Geometry: final body of the model. Coordinates: model frame, mm. A direction names the side the tool comes from. Round coordinates to 2 decimals unless told otherwise and drop trailing zeros. Loops run counter-clockwise (first coordinate to the right, second up) from the corner with the lowest first, then second, coordinate; pieces in that order, holes last. Notation, with made-up numbers: (-5, -13) - (31, -13) arc R16 cw to (31, 18) - close; hole circle Ø3 at (85, -19). An arc over 180 degrees is marked (long way). Answer as CSV lines item,"result".
from build123d import *

# Parameters (mm, degrees)
SKETCH1_R           = 0.899918091
SKETCH1_R_2         = 0.899925125
SKETCH1_R_3         = 1.45
SKETCH1_R_4         = 8
SKETCH1_W           = 3.400011
SKETCH1_H           = 6.2
SKETCH1_W_2         = 3.4
BOSS_EXTRUDE2_DEPTH = 5.85


with BuildPart() as part:
    # Sketch1 → Boss-Extrude2 (new body)
    with BuildSketch(Plane.XY):
        with BuildLine():
            Line((669.21684417, 349.14615334), (647.916445931, 349.14615334))
            ThreePointArc((647.916445931, 349.14615334), (647.089176563, 348.803487148), (646.746510371, 347.976217781))
            Line((646.746510371, 347.976217781), (646.746510371, 315.835342781))
            add(Edge.make_bspline(
                [(646.746510371, 315.835342781), (646.746510371, 314.02716752), (648.773268796, 314.14615334)],
                knots=[0, 0, 0, 1, 1, 1], degree=2))
            Line((648.773268796, 314.14615334), (669.21684417, 314.14615334))
            Line((669.21684417, 314.14615334), (683.493527466, 314.14615334))
            ThreePointArc((683.493527466, 314.14615334), (688.18557682, 319.867900287), (681.655729571, 323.348533873))
            ThreePointArc((681.655729571, 323.348533873), (669.218799175, 331.833597772), (681.99878285, 339.792590441))
            ThreePointArc((681.99878285, 339.792590441), (688.860665305, 343.178948939), (684.070537296, 349.14615334))
            Line((684.070537296, 349.14615334), (669.21684417, 349.14615334))
        make_face()
        with Locations((684.726521371, 342.89615334)):
            Circle(SKETCH1_R, mode=Mode.SUBTRACT)
        with Locations((684.726521371, 320.39615334)):
            Circle(SKETCH1_R_2, mode=Mode.SUBTRACT)
        with Locations((658.726521371, 319.24615334)):
            Circle(SKETCH1_R_3, mode=Mode.SUBTRACT)
        with Locations((658.726521371, 331.64615334)):
            Circle(SKETCH1_R_4, mode=Mode.SUBTRACT)
        with Locations((651.446515871, 343.04615334)):
            Rectangle(SKETCH1_W, SKETCH1_H, mode=Mode.SUBTRACT)
        with Locations((653.576521371, 319.24615334)):
            Rectangle(SKETCH1_W_2, SKETCH1_H, mode=Mode.SUBTRACT)
        with Locations((666.006526871, 343.04615334)):
            Rectangle(SKETCH1_W, SKETCH1_H, mode=Mode.SUBTRACT)
        with Locations((663.876521371, 319.24615334)):
            Rectangle(SKETCH1_W_2, SKETCH1_H, mode=Mode.SUBTRACT)
    extrude(amount=BOSS_EXTRUDE2_DEPTH)


solid = part.part
(1) Access query for faces 1 (the face through (651, 346.146, 3)), 2 (the face through (668, 332, 0)). Directions: +Z, -Z, +X, -X, +Y, -Y. A direction counts if a zero-diameter tool reaches every point of the face in a straight line with its end or side. Return the directions, or none.
Findings below:
face 1,"+Z, -Z"
face 2,"-Z, +X, -X, +Y, -Y"
(2) Section C-C (x = 654). Output: boundary loops of the cut face in (y, z), and give its area (3 significant figures).
Findings below:
outline,"(314.15, 0) - (316.15, 0) - (316.15, 5.85) - (314.15, 5.85) - close; (322.35, 0) - (325.19, 0) - (325.19, 5.85) - (322.35, 5.85) - close; (338.1, 0) - (349.15, 0) - (349.15, 5.85) - (338.1, 5.85) - close"
area,"93.0 mm2"
(3) Pin query (flat end, axial travel): P1, Ø1.5, axis at x = 658.5, z = 3.5, coming from the -Y side; P2, Ø3, axis at y = 333.5, z = 5, coming from the +X side; P3, Ø3, axis at y = 320.5, z = 3.5, coming from the +X side; P4, Ø2.5, axis at x = 658.73, y = 319.25, coming from the +Z side. Return the tip coordinate at first contact, or that it passes through.
Findings below:
P1,"y = 314.15"
P2,"x = 669.87"
P3,"x = 688.28"
P4,"through"
(4) Section D-D (y = 318.5). Output: boundary loops of the cut face in (x, z), and give its area (3 significant figures).
Findings below:
outline,"(646.75, 0) - (651.88, 0) - (651.88, 5.85) - (646.75, 5.85) - close; (655.28, 0) - (657.48, 0) - (657.48, 5.85) - (655.28, 5.85) - close; (659.97, 0) - (662.18, 0) - (662.18, 5.85) - (659.97, 5.85) - close; (665.58, 0) - (688.26, 0) - (688.26, 5.85) - (665.58, 5.85) - close"
area,"189 mm2"
(5) Material intervals for line 1 along X through (y, z) = (318, 2.85); line 2 along X through (y, z) = (317, 0.75); line 3 along Y through (x, z) = (667.5, 5.6), sorted ascending.
Findings below:
line 1,"646.75 to 651.88, 655.28 to 657.99, 659.47 to 662.18, 665.58 to 688.19"
line 2,"646.75 to 651.88, 655.28 to 662.18, 665.58 to 687.87"
line 3,"314.15 to 339.95, 346.15 to 349.15"
(6) Draft query along Y for faces 3 (the face through (653.147, 343, 3)), 4 (the face through (646.747, 332, 3)). Return one class per face: pulls with the +Y half, pulls with the -Y half, needs draft (parallel to the pull), parting line crosses it, or undercut.
Findings below:
face 3,"undercut"
face 4,"needs draft"
(7) Section B-B (x = 675). Output: boundary loops of the cut face in (y, z).
Findings below:
outline,"(314.15, 0) - (323.25, 0) - (323.25, 5.85) - (314.15, 5.85) - close; (340.04, 0) - (349.15, 0) - (349.15, 5.85) - (340.04, 5.85) - close"
(8) Section A-A (y = 333). Output: boundary loops of the cut face in (x, z), and give its area (3 significant figures).
Findings below:
outline,"(646.75, 0) - (650.84, 0) - (650.84, 5.85) - (646.75, 5.85) - close; (666.61, 0) - (669.32, 0) - (669.32, 5.85) - (666.61, 5.85) - close"
area,"39.8 mm2"
